Verification items for the finished model (mm, model axes). Coordinates: 2 decimals unless noted, no trailing zeros. Order: outer loops, then holes, each group sorted by start corner. A loop starts at its lowest first (then second) coordinate and runs counter-clockwise, first axis right, second up. Notation, with made-up numbers: M 76,34.25 L 131,34.25 A20 cw 131,62.25 Z; hole C -35.75,-0.75 d5. An arc over 180 degrees is marked long. Use one line per item in the form item = value. Start each with the question number.
```python
from build123d import *

# Parameters (mm, degrees)
SKETCH1_W             = 70
SKETCH1_H             = 30
SKETCH1_R             = 6.9977
SKETCH1_R_2           = 1.4986
SKETCH1_R_3           = 0.9906
BOSS_EXTRUDE2_DEPTH   = 3.175
F_2_56_TAPPED_HOLE1_D = 1.778
SKETCH4_R             = 3.175
CUT_EXTRUDE1_DEPTH    = 77.223884872


with BuildPart() as part:
    # Sketch1 → Boss-Extrude2 (new body)
    with BuildSketch(Plane.XY):
        with Locations((35, 15)):
            Rectangle(SKETCH1_W, SKETCH1_H)
        with Locations((55, 15)):
            Circle(SKETCH1_R, mode=Mode.SUBTRACT)
        with Locations((37.166699296, 13)):
            Circle(SKETCH1_R_2, mode=Mode.SUBTRACT)
        with Locations((25.169778966, 20.933400182)):
            Circle(SKETCH1_R_3, mode=Mode.SUBTRACT)
    extrude(amount=BOSS_EXTRUDE2_DEPTH)

    # #2-56 Tapped Hole1 (through all)
    with Locations(Plane.XY.offset(3.175)):
        with Locations((67, 27), (67, 3), (3, 27), (3, 3)):
            Hole(F_2_56_TAPPED_HOLE1_D / 2)

    # Sketch4 → Cut-Extrude1 (cut, through all)
    with BuildSketch(Plane.XY.offset(3.175)):
        with Locations((24.0438, 15)):
            Circle(SKETCH4_R)
    extrude(amount=-CUT_EXTRUDE1_DEPTH, mode=Mode.SUBTRACT)


solid = part.part
```
1. Cross-section at B-B on y = 3. Enter the section's corners in (x, z) (3 decimals).
2. Release check for a two-part mould opening along Y. For faces 1 (the flat face through (35, 15, 0)), 2 (the flat face through (35, 30, 2)), 3 (the cylindrical face through (37.972, 14.264, 1.565)) record: pulls with the +Y half, pulls with the -Y half, needs draft (parallel to the pull), parting line crosses it, or undercut.
3. Depth check by flat-ended pin: P1, Ø1.4, axis at x = 3, y = 3, coming from the -Z side. Enter the tip coordinate at first touch or a pass-through.
4. Cross-section at C-C on y = 13. Enter the section's corners in (x, z) (3 decimals).
5. Cross-section at A-A on x = 67. Enter the section's corners in (y, z) (3 decimals), and give its area (3 significant figures).
6. Material ranges on line 1 along Y through (x, z) = (67, 2.45); line 2 along X through (y, z) = (16, 2); line 3 along X through (y, z) = (13.75, 1.85), recorded low to high.
7. Cross-section at D-D on z = 1.95. Give the number of separate pieces and of enclosed holes in the cut face, and give its area (3 significant figures).
Final values:
q1.outline = M 0,0 L 2.111,0 L 2.111,3.175 L 0,3.175 Z; M 3.889,0 L 66.111,0 L 66.111,3.175 L 3.889,3.175 Z; M 67.889,0 L 70,0 L 70,3.175 L 67.889,3.175 Z
q2.face_1 = needs draft
q2.face_2 = pulls with the +Y half
q2.face_3 = undercut
q3.P1 = through
q4.outline = M 0,0 L 21.578,0 L 21.578,3.175 L 0,3.175 Z; M 26.51,0 L 35.668,0 L 35.668,3.175 L 26.51,3.175 Z; M 38.665,0 L 48.294,0 L 48.294,3.175 L 38.665,3.175 Z; M 61.706,0 L 70,0 L 70,3.175 L 61.706,3.175 Z
q5.outline = M 0,0 L 2.111,0 L 2.111,3.175 L 0,3.175 Z; M 3.889,0 L 26.111,0 L 26.111,3.175 L 3.889,3.175 Z; M 27.889,0 L 30,0 L 30,3.175 L 27.889,3.175 Z
q5.area = 84.0 mm2
q6.line_1 = 0 to 2.11, 3.89 to 26.11, 27.89 to 30
q6.line_2 = 0 to 21.03, 27.06 to 48.07, 61.93 to 70
q6.line_3 = 0 to 21.13, 26.96 to 35.87, 38.46 to 48.11, 61.89 to 70
q7.separate_pieces = 1
q7.enclosed_holes = 8
q7.area = 1,890 mm2
